Source: CAD feature listing. Evaluate the final solid. Frame: model axes, mm. A direction names the side the tool comes from. Give positions to 0.01 mm unless a question says otherwise; leave off trailing zeros. Order: outer loops, then holes, each group sorted by start corner. A loop starts at its lowest first (then second) coordinate and runs counter-clockwise, first axis right, second up. Notation, with made-up numbers: (33, -22.75) - (59, -22.75) arc R17 cw to (59, 9.25) - close; hole circle Ø1 at (-10.75, 48.5). An arc over 180 degrees is marked (long way). Use CSV: the item, a comma, the result in double quotes.
```python
from build123d import *

# Parameters (mm, degrees)
SKETCH1_W           = 22
SKETCH1_H           = 55
SKETCH1_R           = 5.25
SKETCH1_W_2         = 4
SKETCH1_H_2         = 2.5
BOSS_EXTRUDE1_DEPTH = 18
SKETCH2_R           = 5.25
CUT_EXTRUDE1_DEPTH  = 23
SKETCH3_R           = 4
CUT_EXTRUDE2_DEPTH  = 20
CHAMFER1_SIZE       = 2
SKETCH4_R           = 11
CUT_EXTRUDE3_DEPTH  = 2
FILLET1_R           = 1
CHAMFER2_SIZE       = 2


with BuildPart() as part:
    # Sketch1 → Boss-Extrude1 (new body)
    with BuildSketch(Plane.XY):
        with Locations((11, 27.5)):
            Rectangle(SKETCH1_W, SKETCH1_H)
        with Locations((11, 12)):
            Circle(SKETCH1_R, mode=Mode.SUBTRACT)
        with Locations((11, 34)):
            Circle(SKETCH1_R, mode=Mode.SUBTRACT)
        with Locations((11, 45)):
            Rectangle(SKETCH1_W_2, SKETCH1_H_2, mode=Mode.SUBTRACT)
    extrude(amount=-BOSS_EXTRUDE1_DEPTH)

    # Sketch2 → Cut-Extrude1 (cut, through all)
    with BuildSketch(Plane.ZY):
        with Locations((-9, 23)):
            Circle(SKETCH2_R)
    extrude(amount=-CUT_EXTRUDE1_DEPTH, mode=Mode.SUBTRACT)

    # Sketch3 → Cut-Extrude2 (cut)
    with BuildSketch(Plane(origin=(0, 0, 0), x_dir=(0, 0, -1), z_dir=(1, 0, 0))):
        with Locations((9, 53.5)):
            Circle(SKETCH3_R)
    extrude(amount=CUT_EXTRUDE2_DEPTH, mode=Mode.SUBTRACT)

    # Chamfer1
    chamfer1_edges = [part.edges().sort_by_distance(p)[0] for p in [
        (22, 27.5, 0),
        (22, 27.5, -18),
    ]]
    chamfer(chamfer1_edges, length=CHAMFER1_SIZE)

    # Sketch4 → Cut-Extrude3 (cut)
    with BuildSketch(Plane(origin=(22, 0, 0), x_dir=(0, 0, -1), z_dir=(1, 0, 0))):
        with Locations((9, 23)):
            Circle(SKETCH4_R)
    extrude(amount=-CUT_EXTRUDE3_DEPTH, mode=Mode.SUBTRACT)

    # Fillet1
    fillet1_edges = [part.edges().sort_by_distance(p)[0] for p in [
        (22, 34, -9),
        (22, 12, -9),
    ]]
    fillet(fillet1_edges, radius=FILLET1_R)

    # Chamfer2
    chamfer2_edges = [part.edges().sort_by_distance(p)[0] for p in [
        (10, 55, 0),
        (10, 55, -18),
    ]]
    chamfer(chamfer2_edges, length=CHAMFER2_SIZE)


solid = part.part
```
Item 1: Section D-D on y = 53.5. Return the cut outline in (x, z), then the cut area to 3 significant figures.
Filled in:
outline,"(0, -17.5) - (20.5, -17.5) - (22, -16) - (22, -2) - (20.5, -0.5) - (0, -0.5) - (0, -5) - (20, -5) - (20, -13) - (0, -13) - close"
area,"212 mm2"
Item 2: Set-up query: faces 4 (the flat face through (21, 8, -17)), 5 (the cylindrical face through (20.5, 12, -8.9)), 6 (the flat face through (11, 46.25, -9)). Return all of +Z, -Z, +X, -X, +Y, -Y with unobstructed straight access to the full face (end or side cutting, diameter ignored); none if empty.
Filled in:
face 4,"-Z, +X, +Y, -Y"
face 5,"+X"
face 6,"+Z, -Z"
Item 3: Section C-C on y = 8.5. Return the cut outline in (x, z).
Filled in:
outline,"(0, -18) - (7.09, -18) - (7.09, 0) - (0, 0) - close; (14.91, -18) - (20, -18) - (22, -16) - (22, -2) - (20, 0) - (14.91, 0) - close"
Item 4: Material intervals for line 1 (Y direction, x = 13.75, z = -10.5); line 2 (Y direction, x = 10, z = -16); line 3 (Y direction, x = 11, z = -5.5), sorted ascending. Write a range as from..to.
Filled in:
line 1,"y = 0..7.53, 16.47..17.97, 28.03..29.53, 38.47..49.79"
line 2,"y = 0..6.85, 17.15..28.85, 39.15..43.75, 46.25..55"
line 3,"y = 0..6.75, 17.25..19.09, 26.91..28.75, 39.25..43.75, 46.25..51.56"
Item 5: Section A-A on z = -9. Return the cut outline in (x, y).
Filled in:
outline,"(0, 0) - (22, 0) - (22, 11) arc R1 ccw to (21, 12) - (20, 12) - (20, 17.75) - (0, 17.75) - close; (0, 28.25) - (20, 28.25) - (20, 34) - (21, 34) arc R1 ccw to (22, 35) - (22, 55) - (20, 55) - (20, 49.5) - (0, 49.5) - close; hole circle Ø10.5 at (11, 12); hole circle Ø10.5 at (11, 34); hole (9, 43.75) - (13, 43.75) - (13, 46.25) - (9, 46.25) - close"
Item 6: Mould query, pull axis Z, two halves, no side actions, for faces 1 (the flat face through (21, 42, -1)), 2 (the flat face through (22, 7, -9)), 3 (the cylindrical face through (9.9, 49.5, -8.9)). Classes: released by +Z, released by -Z, zero draft, split by the parting line, or undercut.
Filled in:
face 1,"released by +Z"
face 2,"zero draft"
face 3,"undercut"
Item 7: Section B-B on x = 13.5. Return the cut outline in (y, z), then the cut area to 3 significant figures.
Filled in:
outline,"(0, -18) - (7.38, -18) - (7.38, 0) - (0, 0) - close; (16.62, -18) - (29.38, -18) - (29.38, 0) - (16.62, 0) - close; (38.62, -18) - (53, -18) - (55, -16) - (55, -12.71) arc R4 cw (long way) to (55, -5.29) - (55, -2) - (53, 0) - (38.62, 0) - close; hole circle Ø10.5 at (23, -9)"
area,"530 mm2"
